Design review of the part built by this model. Coordinates are the model's own, in mm. Face numbers are marked on the shaded views. A direction names the side the tool comes from. Give positions to 0.01 mm unless a question says otherwise; leave off trailing zeros. Order: outer loops, then holes, each group sorted by start corner. A loop starts at its lowest first (then second) coordinate and runs counter-clockwise, first axis right, second up. Notation, with made-up numbers: (39, -20.75) -> (47, -20.75) arc R18 cw to (47, 2.25) -> close; hole circle Ø6 at (49.25, -9). An arc over 180 degrees is marked (long way). One line per item, written item: value. Start each with the question number.
1) Consider section B-B (y = 60). State the section outline as (x, z) points, plus the area to 3 significant figures.
2) Tool access review of the marked faces 4 and 5: name each direction out of +Z, -Z, +X, -X, +Y, -Y from which nothing blocks a thin tool from reaching the whole face with its end or side.
3) The part is to be moulded in two halves that separate along Y. For the marked faces 1, 2 and 3, say which applies: released by +Y, released by -Y, zero draft, split by the parting line, or undercut.
4) Consider section D-D (x = -85). State the section outline as (y, z) points, plus the area to 4 significant figures.
5) For pin 1 (4 mm diameter, centred on x = -138, y = 10, fed in from +Z); pin 2 (8 mm diameter, centred on x = -54, y = 11, fed in from +Z); pin 3 (23 mm diameter, centred on x = -61, y = 28.5, fed in from -Z); pin 4 (4 mm diameter, centred on y = 62.5, z = -22.5, fed in from -X), all flat-tipped, find the tip position at first contact; note any pin that passes through.
6) Consider section A-A (x = -137.5). State the section outline as (y, z) points.
7) Consider section C-C (z = -17). State the section outline as (x, y) points, plus the area to 3 significant figures.
8) Wall thickness on line 1 along Y through (x, z) = (-39, -0.6); line 2 along Y through (x, z) = (-111.5, -78); line 3 along Z through (x, y) = (-112.5, 18): over which ranges is each line inside the solid? List them lowest first. Write a range as from..to.
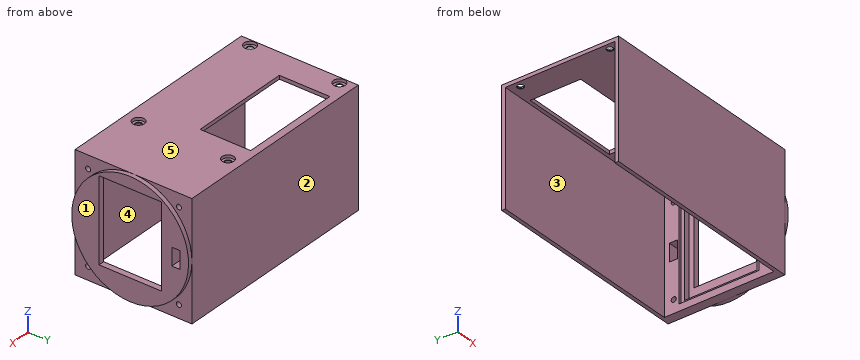
from build123d import *

# Parameters (mm, degrees)
SZKIC1_R                    = 40.5
SZKIC1_W                    = 57.6
SZKIC1_H                    = 43.2
DODANIE_WYCI_GNI_CIE1_DEPTH = 8
DODANIE_WYCI_GNI_CIE2_DEPTH = 5
SZKIC2_W                    = 69.32
SZKIC2_H                    = 50.12
SZKIC2_W_2                  = 57.6
SZKIC2_H_2                  = 43.2
WYTNIJ_WYCI_GNI_CIE1_DEPTH  = 3.9
SZKIC2_4_W                  = 81
SZKIC2_4_H                  = 81
SZKIC2_4_W_2                = 73.3
SZKIC2_4_H_2                = 55.32
DODANIE_WYCI_GNI_CIE3_DEPTH = 2
DODANIE_WYCI_GNI_CIE4_DEPTH = 140
WYTNIJ_WYCI_GNI_CIE2_REACH  = 184.445
SZKIC5_R                    = 2.25
SZKIC6_R                    = 4.1
WYTNIJ_WYCI_GNI_CIE3_DEPTH  = 2
WYTNIJ_WYCI_GNI_CIE4_REACH  = 184.445
SZKIC7_W                    = 70
SZKIC7_H                    = 35
WYTNIJ_WYCI_GNI_CIE5_REACH  = 188.363
SZKIC8_R                    = 1.75
WYTNIJ_WYCI_GNI_CIE6_REACH  = 190.738
SZKIC9_W                    = 12.2
SZKIC9_H                    = 5.6
SZKIC10_W                   = 140
SZKIC10_H                   = 78
WYTNIJ_WYCI_GNI_CIE7_DEPTH  = 0.5
SZKIC11_W                   = 140
SZKIC11_H                   = 78
WYTNIJ_WYCI_GNI_CIE8_DEPTH  = 0.5
WYTNIJ_WYCI_GNI_CIE9_DEPTH  = 0.5
WYTNIJ_WYCI_GNI_CIE10_DEPTH = 0.5


with BuildPart() as part:
    # Szkic1 → Dodanie-wyci_gni_cie1 (new body)
    with BuildSketch(Plane(origin=(0, 0, 0), x_dir=(0, 0, -1), z_dir=(1, 0, 0))):
        with Locations((40.5, 40.5)):
            Circle(SZKIC1_R)
        with Locations((36.8, 40.5)):
            Rectangle(SZKIC1_W, SZKIC1_H, mode=Mode.SUBTRACT)
    extrude(amount=DODANIE_WYCI_GNI_CIE1_DEPTH)

    # Szkic1_3 → Dodanie-wyci_gni_cie2 (add)
    with BuildSketch(Plane(origin=(0, 0, 0), x_dir=(0, 0, -1), z_dir=(1, 0, 0))):
        with BuildLine():
            Line((40.5, 81), (0, 81))
            Line((0, 81), (0, 40.5))
            ThreePointArc((0, 40.5), (11.862175362, 69.137824638), (40.5, 81))
        make_face()
        with BuildLine():
            Line((81, 81), (40.5, 81))
            ThreePointArc((40.5, 81), (69.137824638, 69.137824638), (81, 40.5))
            Line((81, 40.5), (81, 81))
        make_face()
        with BuildLine():
            Line((81, 0), (81, 40.5))
            ThreePointArc((81, 40.5), (69.137824638, 11.862175362), (40.5, 0))
            Line((40.5, 0), (81, 0))
        make_face()
        with BuildLine():
            ThreePointArc((40.5, 0), (11.862175362, 11.862175362), (0, 40.5))
            Line((0, 40.5), (0, 0))
            Line((0, 0), (40.5, 0))
        make_face()
    extrude(amount=DODANIE_WYCI_GNI_CIE2_DEPTH)

    # Szkic2 → Wytnij-wyci_gni_cie1 (cut)
    with BuildSketch(Plane.ZY):
        with Locations((-39.6, 40.5)):
            Rectangle(SZKIC2_W, SZKIC2_H)
        with Locations((-36.8, 40.5)):
            Rectangle(SZKIC2_W_2, SZKIC2_H_2, mode=Mode.SUBTRACT)
    extrude(amount=-WYTNIJ_WYCI_GNI_CIE1_DEPTH, mode=Mode.SUBTRACT)

    # Szkic2_4 → Dodanie-wyci_gni_cie3 (add)
    with BuildSketch(Plane.ZY):
        with Locations((-40.5, 40.5)):
            Rectangle(SZKIC2_4_W, SZKIC2_4_H)
        with Locations((-39.65, 40.5)):
            Rectangle(SZKIC2_4_W_2, SZKIC2_4_H_2, mode=Mode.SUBTRACT)
    extrude(amount=DODANIE_WYCI_GNI_CIE3_DEPTH)

    # Szkic3 → Dodanie-wyci_gni_cie4 (add)
    with BuildSketch(Plane.ZY.offset(2)):
        Polygon((-81, 0), (0, 0), (0, 81), (-81, 81), (-81, 78), (-3, 78), (-3, 3), (-81, 3), align=None)
    extrude(amount=DODANIE_WYCI_GNI_CIE4_DEPTH)

    # Szkic5 → Wytnij-wyci_gni_cie2 (cut, up to next)
    with BuildSketch(Plane.XY, mode=Mode.PRIVATE) as wytnij_wyci_gni_cie2_sk1:
        with Locations((-137.5, 71.5)):
            Circle(SZKIC5_R)
    wytnij_wyci_gni_cie2_tool1 = extrude(wytnij_wyci_gni_cie2_sk1.sketch, amount=-WYTNIJ_WYCI_GNI_CIE2_REACH, mode=Mode.PRIVATE) & part.part
    # Szkic5 → Wytnij-wyci_gni_cie2 (cut, up to next)
    with BuildSketch(Plane.XY, mode=Mode.PRIVATE) as wytnij_wyci_gni_cie2_sk2:
        with Locations((-39, 71.5)):
            Circle(SZKIC5_R)
    wytnij_wyci_gni_cie2_tool2 = extrude(wytnij_wyci_gni_cie2_sk2.sketch, amount=-WYTNIJ_WYCI_GNI_CIE2_REACH, mode=Mode.PRIVATE) & part.part
    # Szkic5 → Wytnij-wyci_gni_cie2 (cut, up to next)
    with BuildSketch(Plane.XY, mode=Mode.PRIVATE) as wytnij_wyci_gni_cie2_sk3:
        with Locations((-137.5, 9.5)):
            Circle(SZKIC5_R)
    wytnij_wyci_gni_cie2_tool3 = extrude(wytnij_wyci_gni_cie2_sk3.sketch, amount=-WYTNIJ_WYCI_GNI_CIE2_REACH, mode=Mode.PRIVATE) & part.part
    # Szkic5 → Wytnij-wyci_gni_cie2 (cut, up to next)
    with BuildSketch(Plane.XY, mode=Mode.PRIVATE) as wytnij_wyci_gni_cie2_sk4:
        with Locations((-39, 9.5)):
            Circle(SZKIC5_R)
    wytnij_wyci_gni_cie2_tool4 = extrude(wytnij_wyci_gni_cie2_sk4.sketch, amount=-WYTNIJ_WYCI_GNI_CIE2_REACH, mode=Mode.PRIVATE) & part.part
    add(wytnij_wyci_gni_cie2_tool1.solids().sort_by_distance((-137.5, 71.5, 0))[0], mode=Mode.SUBTRACT)
    add(wytnij_wyci_gni_cie2_tool2.solids().sort_by_distance((-39, 71.5, 0))[0], mode=Mode.SUBTRACT)
    add(wytnij_wyci_gni_cie2_tool3.solids().sort_by_distance((-137.5, 9.5, 0))[0], mode=Mode.SUBTRACT)
    add(wytnij_wyci_gni_cie2_tool4.solids().sort_by_distance((-39, 9.5, 0))[0], mode=Mode.SUBTRACT)

    # Szkic6 → Wytnij-wyci_gni_cie3 (cut)
    with BuildSketch(Plane.XY):
        with Locations((-137.5, 71.5)):
            Circle(SZKIC6_R)
        with Locations((-39, 71.5)):
            Circle(SZKIC6_R)
        with Locations((-39, 9.5)):
            Circle(SZKIC6_R)
        with Locations((-137.5, 9.5)):
            Circle(SZKIC6_R)
    extrude(amount=-WYTNIJ_WYCI_GNI_CIE3_DEPTH, mode=Mode.SUBTRACT)

    # Szkic7 → Wytnij-wyci_gni_cie4 (cut, up to next)
    with BuildSketch(Plane.XY, mode=Mode.PRIVATE) as wytnij_wyci_gni_cie4_sk1:
        with Locations((-88.25, 58.5)):
            Rectangle(SZKIC7_W, SZKIC7_H)
    wytnij_wyci_gni_cie4_tool1 = extrude(wytnij_wyci_gni_cie4_sk1.sketch, amount=-WYTNIJ_WYCI_GNI_CIE4_REACH, mode=Mode.PRIVATE) & part.part
    add(wytnij_wyci_gni_cie4_tool1.solids().sort_by_distance((-88.25, 58.5, 0))[0], mode=Mode.SUBTRACT)

    # Szkic8 → Wytnij-wyci_gni_cie5 (cut, up to next)
    with BuildSketch(Plane(origin=(5, 0, 0), x_dir=(0, 0, -1), z_dir=(1, 0, 0)), mode=Mode.PRIVATE) as wytnij_wyci_gni_cie5_sk1:
        with Locations((9.033748237, 71.966251763)):
            Circle(SZKIC8_R)
    wytnij_wyci_gni_cie5_tool1 = extrude(wytnij_wyci_gni_cie5_sk1.sketch, amount=-WYTNIJ_WYCI_GNI_CIE5_REACH, mode=Mode.PRIVATE) & part.part
    # Szkic8 → Wytnij-wyci_gni_cie5 (cut, up to next)
    with BuildSketch(Plane(origin=(5, 0, 0), x_dir=(0, 0, -1), z_dir=(1, 0, 0)), mode=Mode.PRIVATE) as wytnij_wyci_gni_cie5_sk2:
        with Locations((71.966251763, 71.966251763)):
            Circle(SZKIC8_R)
    wytnij_wyci_gni_cie5_tool2 = extrude(wytnij_wyci_gni_cie5_sk2.sketch, amount=-WYTNIJ_WYCI_GNI_CIE5_REACH, mode=Mode.PRIVATE) & part.part
    # Szkic8 → Wytnij-wyci_gni_cie5 (cut, up to next)
    with BuildSketch(Plane(origin=(5, 0, 0), x_dir=(0, 0, -1), z_dir=(1, 0, 0)), mode=Mode.PRIVATE) as wytnij_wyci_gni_cie5_sk3:
        with Locations((71.966251763, 9.033748237)):
            Circle(SZKIC8_R)
    wytnij_wyci_gni_cie5_tool3 = extrude(wytnij_wyci_gni_cie5_sk3.sketch, amount=-WYTNIJ_WYCI_GNI_CIE5_REACH, mode=Mode.PRIVATE) & part.part
    # Szkic8 → Wytnij-wyci_gni_cie5 (cut, up to next)
    with BuildSketch(Plane(origin=(5, 0, 0), x_dir=(0, 0, -1), z_dir=(1, 0, 0)), mode=Mode.PRIVATE) as wytnij_wyci_gni_cie5_sk4:
        with Locations((9.033748237, 9.033748237)):
            Circle(SZKIC8_R)
    wytnij_wyci_gni_cie5_tool4 = extrude(wytnij_wyci_gni_cie5_sk4.sketch, amount=-WYTNIJ_WYCI_GNI_CIE5_REACH, mode=Mode.PRIVATE) & part.part
    add(wytnij_wyci_gni_cie5_tool1.solids().sort_by_distance((5, 71.966252, -9.033748))[0], mode=Mode.SUBTRACT)
    add(wytnij_wyci_gni_cie5_tool2.solids().sort_by_distance((5, 71.966252, -71.966252))[0], mode=Mode.SUBTRACT)
    add(wytnij_wyci_gni_cie5_tool3.solids().sort_by_distance((5, 9.033748, -71.966252))[0], mode=Mode.SUBTRACT)
    add(wytnij_wyci_gni_cie5_tool4.solids().sort_by_distance((5, 9.033748, -9.033748))[0], mode=Mode.SUBTRACT)

    # Szkic9 → Wytnij-wyci_gni_cie6 (cut, up to next)
    with BuildSketch(Plane(origin=(8, 0, 0), x_dir=(0, 0, -1), z_dir=(1, 0, 0)), mode=Mode.PRIVATE) as wytnij_wyci_gni_cie6_sk1:
        with Locations((40.5, 72.2)):
            Rectangle(SZKIC9_W, SZKIC9_H)
    wytnij_wyci_gni_cie6_tool1 = extrude(wytnij_wyci_gni_cie6_sk1.sketch, amount=-WYTNIJ_WYCI_GNI_CIE6_REACH, mode=Mode.PRIVATE) & part.part
    add(wytnij_wyci_gni_cie6_tool1.solids().sort_by_distance((8, 72.2, -40.5))[0], mode=Mode.SUBTRACT)

    # Szkic10 → Wytnij-wyci_gni_cie7 (cut)
    with BuildSketch(Plane.XZ.offset(-78)):
        with Locations((-72, -42)):
            Rectangle(SZKIC10_W, SZKIC10_H)
    extrude(amount=-WYTNIJ_WYCI_GNI_CIE7_DEPTH, mode=Mode.SUBTRACT)

    # Szkic11 → Wytnij-wyci_gni_cie8 (cut)
    with BuildSketch(Plane(origin=(0, 3, 0), x_dir=(1, 0, 0), z_dir=(0, 1, 0))):
        with Locations((-72, 42)):
            Rectangle(SZKIC11_W, SZKIC11_H)
    extrude(amount=-WYTNIJ_WYCI_GNI_CIE8_DEPTH, mode=Mode.SUBTRACT)

    # Szkic12 → Wytnij-wyci_gni_cie9 (cut)
    with BuildSketch(Plane.ZY.offset(2)):
        Polygon((-81, 78.5), (-81, 2.5), (-3, 2.5), (-3, 12.84), (-76.3, 12.84), (-76.3, 68.16), (-3, 68.16), (-3, 78.5), align=None)
    extrude(amount=-WYTNIJ_WYCI_GNI_CIE9_DEPTH, mode=Mode.SUBTRACT)

    # Szkic13 → Wytnij-wyci_gni_cie10 (cut)
    with BuildSketch(Plane(origin=(0, 0, -3), x_dir=(-1, 0, 0), z_dir=(0, 0, -1))):
        Polygon((1.5, 78.5), (1.5, 68.16), (0, 68.16), (0, 12.84), (1.5, 12.84), (1.5, 2.5), (142, 2.5), (142, 78.5), align=None)
    extrude(amount=-WYTNIJ_WYCI_GNI_CIE10_DEPTH, mode=Mode.SUBTRACT)


solid = part.part
Checked values:
1. outline: (-142, -2.5) -> (-123.25, -2.5) -> (-123.25, 0) -> (-142, 0) -> close; (-53.25, -2.5) -> (0, -2.5) -> (0, -4.94) -> (3.9, -4.94) -> (3.9, -8) -> (8, -8) -> (8, -5) -> (5, -5) -> (5, 0) -> (-53.25, 0) -> close; (-1.5, -81) -> (5, -81) -> (5, -76) -> (8, -76) -> (8, -65.6) -> (3.9, -65.6) -> (3.9, -74.26) -> (0, -74.26) -> (0, -76.3) -> (-1.5, -76.3) -> close
1. area: 299 mm^2
2. face 4: -Z, -X
2. face 5: +Z, +X, -X, +Y, -Y
3. face 1: zero draft
3. face 2: released by +Y
3. face 3: undercut
4. outline: (0, -81) -> (2.5, -81) -> (2.5, -2.5) -> (41, -2.5) -> (41, 0) -> (0, 0) -> close; (76, -2.5) -> (78.5, -2.5) -> (78.5, -81) -> (81, -81) -> (81, 0) -> (76, 0) -> close
4. area: 507.5 mm^2
5. pin 1: stops at z = -2
5. pin 2: stops at z = 0
5. pin 3: stops at z = -2.5
5. pin 4: stops at x = 3.9
6. outline: (0, -81) -> (2.5, -81) -> (2.5, -2.5) -> (7.25, -2.5) -> (7.25, -2) -> (5.4, -2) -> (5.4, 0) -> (0, 0) -> close; (11.75, -2.5) -> (69.25, -2.5) -> (69.25, -2) -> (67.4, -2) -> (67.4, 0) -> (13.6, 0) -> (13.6, -2) -> (11.75, -2) -> close; (73.75, -2.5) -> (78.5, -2.5) -> (78.5, -81) -> (81, -81) -> (81, 0) -> (75.6, 0) -> (75.6, -2) -> (73.75, -2) -> close
7. outline: (-142, 0) -> (5, 0) -> (5, 7.52) -> (8, 7.52) -> (8, 18.9) -> (3.9, 18.9) -> (3.9, 15.44) -> (0, 15.44) -> (0, 12.84) -> (-1.5, 12.84) -> (-1.5, 2.5) -> (-142, 2.5) -> close; (-142, 78.5) -> (-1.5, 78.5) -> (-1.5, 68.16) -> (0, 68.16) -> (0, 65.56) -> (3.9, 65.56) -> (3.9, 62.1) -> (8, 62.1) -> (8, 73.48) -> (5, 73.48) -> (5, 81) -> (-142, 81) -> close
7. area: 971 mm^2
8. line 1: y = 0..5.4, 13.6..67.4, 75.6..81
8. line 2: y = 0..2.5, 78.5..81
8. line 3: z = -2.5..0
